Part print with two shaded views. Sizes in mm from the minimum x, y, z corner. Round coordinates to 2 decimals unless told otherwise and drop trailing zeros. Write each loop counter-clockwise with the first axis right and the second up, starting at its lowest first coordinate (ties: lowest second). Pieces come first, ordered by that corner, then holes. Notation, with made-up numbers: M 61,-34 L 80,-34 A21 cw 80,-7 Z; hole C 47.5,34.25 d1. An arc over 180 degrees is marked long. One line per question, with ' | ' between items. Start each with the question number.
1) Saw through at C-C (y = 4). List the corners of the cut face in (x, z), plus the area to 3 significant figures.
2) Saw through at A-A (x = 40). List the corners of the cut face in (y, z), plus the area to 3 significant figures.
3) Wall check: probe 1 along Z at (x, y) = (40, 4.5); probe 2 along X at (y, z) = (5.5, 48.5); probe 3 along Z at (x, y) = (34.5, 3.25). Give the ranges that are in metal, low to high. Write a range as [from, to].
4) Mould opens along X. For the marked faces 1, 2, 3 and 4 say: pulls with the +X half, pulls with the -X half, needs draft (parallel to the pull), parting line crosses it, or undercut.
5) Drop a flat-ended pin along its axis: pin 1 Ø12 at (x, z) = (40, 40) entering from -Y. Give the stop position or say it passes through.
6) Saw through at B-B (z = 40). List the corners of the cut face in (x, y).
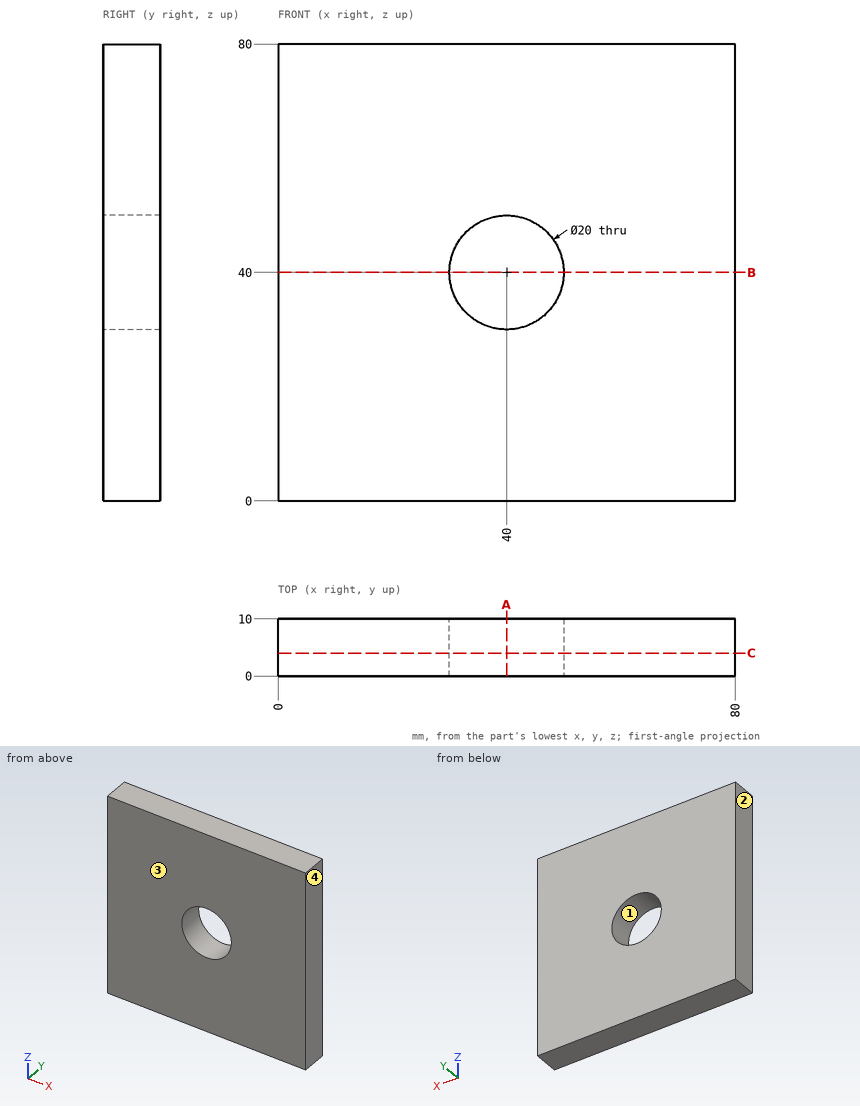
Answer key:
1) outline: M 0,0 L 80,0 L 80,80 L 0,80 Z; hole C 40,40 d20 | area: 6,090 mm2
2) outline: M 0,0 L 10,0 L 10,30 L 0,30 Z; M 0,50 L 10,50 L 10,80 L 0,80 Z | area: 600 mm2
3) probe 1: z = [0, 30], [50, 80] | probe 2: x = [0, 34.73], [45.27, 80] | probe 3: z = [0, 31.65], [48.35, 80]
4) face 1: undercut | face 2: pulls with the -X half | face 3: needs draft | face 4: pulls with the +X half
5) pin 1: passes through
6) outline: M 0,0 L 30,0 L 30,10 L 0,10 Z; M 50,0 L 80,0 L 80,10 L 50,10 Z
